Source: three-view drawing plus pictorial views. Frame: mm from the lowest corner of the part. Give positions to 0.01 mm unless a question says otherwise; leave off trailing zeros. Loops run counter-clockwise (first coordinate to the right, second up) from the corner with the lowest first, then second, coordinate; pieces in that order, holes last. Notation, with made-up numbers: (-25, 37) - (32, 37) arc R7 ccw to (32, 42) - close; hole circle Ø11 at (85.5, 67.5). An arc over 180 degrees is marked (long way). One line per item, written item: value.
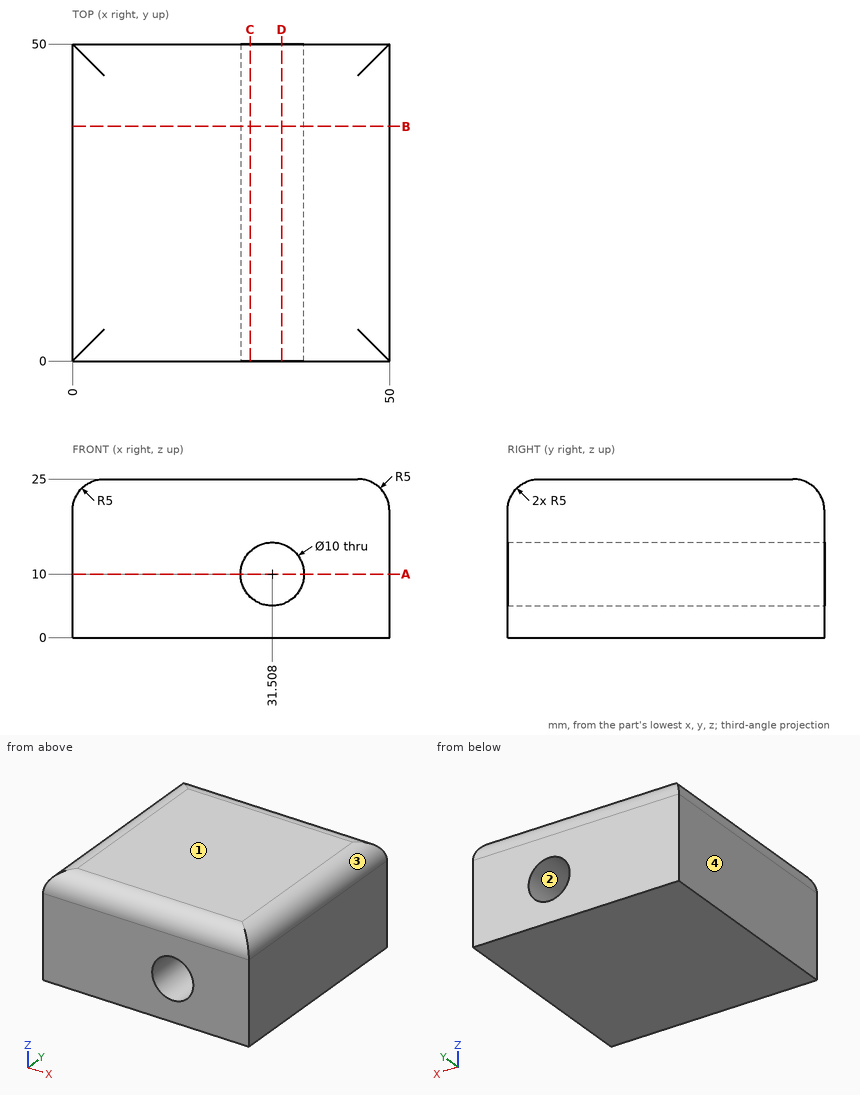
Item 1: Draft query along X for the marked faces 1, 2, 3 and 4. Return one class per face: pulls with the +X half, pulls with the -X half, needs draft (parallel to the pull), parting line crosses it, or undercut.
Verdict:
face 1: needs draft
face 2: undercut
face 3: pulls with the +X half
face 4: pulls with the -X half
Item 2: Section C-C, the plane x = 28. Output: boundary loops of the cut face in (y, z), and give its area (3 significant figures).
Verdict:
outline: (0, 0) - (50, 0) - (50, 6.44) - (0, 6.44) - close; (0, 13.56) - (50, 13.56) - (50, 20) arc R5 ccw to (45, 25) - (5, 25) arc R5 ccw to (0, 20) - close
area: 883 mm^2
Item 3: Pin query (flat end, axial travel): P1, Ø6, axis at x = 5.5, y = 44.5, coming from the -Z side. Return the tip coordinate at first contact, or that it passes through.
Verdict:
P1: stops at z = 0
Item 4: Section D-D, the plane x = 33. Output: boundary loops of the cut face in (y, z), and give its area (3 significant figures).
Verdict:
outline: (0, 0) - (50, 0) - (50, 5.23) - (0, 5.23) - close; (0, 14.77) - (50, 14.77) - (50, 20) arc R5 ccw to (45, 25) - (5, 25) arc R5 ccw to (0, 20) - close
area: 762 mm^2
Item 5: Section A-A, the plane z = 10. Output: boundary loops of the cut face in (x, y), and give its area (3 significant figures).
Verdict:
outline: (0, 0) - (26.51, 0) - (26.51, 50) - (0, 50) - close; (36.51, 0) - (50, 0) - (50, 50) - (36.51, 50) - close
area: 2,000 mm^2
Item 6: Material intervals for L1, parallel to X at y = 26, z = 11.25; L2, parallel to Z at x = 29.5, y = 4; L3, parallel to X at y = 27, z = 12.75 (1 decimal), sorted ascending.
Verdict:
L1: x = 0 to 26.67, 36.35 to 50
L2: z = 0 to 5.42, 14.58 to 24.9
L3: x = 0 to 27.3, 35.7 to 50
Item 7: Section B-B, the plane y = 37. Output: boundary loops of the cut face in (x, z), and give its area (3 significant figures).
Verdict:
outline: (0, 0) - (50, 0) - (50, 20) arc R5 ccw to (45, 25) - (5, 25) arc R5 ccw to (0, 20) - close; hole circle Ø10 at (31.51, 10)
area: 1,160 mm^2
